Design review of the part built by this model. Coordinates are the model's own, in mm. A direction names the side the tool comes from. Give positions to 0.01 mm unless a question says otherwise; leave off trailing zeros. Write each loop counter-clockwise with the first axis right and the second up, starting at its lowest first coordinate (ties: lowest second). Pieces come first, ordered by that corner, then holes. Notation, with made-up numbers: M 78.25,-19.5 L 116.25,-19.5 A31 cw 116.25,19.5 Z; hole C 13,88.5 d3. An arc over 180 degrees is marked long. Answer in a Markdown table with one row per item.
```python
from build123d import *

# Parameters (mm, degrees)
SKETCH_1_R      = 1.1
SKETCH_1_R_2    = 1.6
EXTRUDE_1_DEPTH = 5


with BuildPart() as part:
    # ｽｹｯﾁ1 → ﾎﾞｽ - 押し出し1 (new body)
    with BuildSketch(Plane(origin=(0, 0, 0), x_dir=(1, 0, 0), z_dir=(0, 1, 0))):
        with BuildLine():
            Line((-15.999307359, 14.052631579), (-16.998961039, -23.921052632))
            ThreePointArc((-16.998961039, -23.921052632), (-16.149051198, -26.093222145), (-14, -27))
            Line((-14, -27), (14, -27))
            ThreePointArc((14, -27), (16.149051198, -26.093222145), (16.998961039, -23.921052632))
            Line((16.998961039, -23.921052632), (15.999307359, 14.052631579))
            ThreePointArc((15.999307359, 14.052631579), (15.39548143, 15.432700799), (14, 16))
            Line((14, 16), (-14, 16))
            ThreePointArc((-14, 16), (-15.39548143, 15.432700799), (-15.999307359, 14.052631579))
        make_face()
        with Locations(Location((-14, 14, 0), (0, 0, 270))):
            Circle(SKETCH_1_R, mode=Mode.SUBTRACT)
        with Locations(Location((14, 14, 0), (0, 0, 270))):
            Circle(SKETCH_1_R, mode=Mode.SUBTRACT)
        with Locations(Location((14, -14, 0), (0, 0, 270))):
            Circle(SKETCH_1_R, mode=Mode.SUBTRACT)
        with Locations(Location((-14, -14, 0), (0, 0, 270))):
            Circle(SKETCH_1_R, mode=Mode.SUBTRACT)
        with Locations(Location((-14, -24, 0), (0, 0, 270))):
            Circle(SKETCH_1_R_2, mode=Mode.SUBTRACT)
        with Locations(Location((14, -24, 0), (0, 0, 270))):
            Circle(SKETCH_1_R_2, mode=Mode.SUBTRACT)
        with BuildLine():
            Line((-14, 12), (-14, -12))
            ThreePointArc((-14, -12), (-12.585786438, -12.585786438), (-12, -14))
            Line((-12, -14), (12, -14))
            ThreePointArc((12, -14), (12.585786438, -12.585786438), (14, -12))
            Line((14, -12), (14, 12))
            ThreePointArc((14, 12), (12.585786438, 12.585786438), (12, 14))
            Line((12, 14), (-12, 14))
            ThreePointArc((-12, 14), (-12.585786438, 12.585786438), (-14, 12))
        make_face(mode=Mode.SUBTRACT)
    extrude(amount=EXTRUDE_1_DEPTH)


solid = part.part
```
1) To check wall thickness, follow probe 1 along X at (y, z) = (1.85, 24); probe 2 along Z at (x, y) = (4, 1.6); probe 3 along X at (y, z) = (4, 10). State the ranges of each line that lie inside material, in increasing order. Write a range as [from, to].
Geometry says:
| item | result |
|---|---|
| probe 1 | [-17, -15.6], [-12.4, 12.4], [15.6, 17] |
| probe 2 | [-16, -14], [14, 27] |
| probe 3 | [-16.63, -14], [14, 16.63] |
2) Add section C-C (y = 2.4). Write out the cut boundary in (x, z).
Geometry says:
| item | result |
|---|---|
| outline | M -17,23.92 L -16,-14.05 A2 ccw -14,-16 L 14,-16 A2 ccw 16,-14.05 L 17,23.92 A3 ccw 14,27 L -14,27 A3 ccw Z; hole C -14,24 d3.2; hole C -14,-14 d2.2; hole C -14,14 d2.2; hole M -14,-12 A2 cw -12,-14 L 12,-14 A2 cw 14,-12 L 14,12 A2 cw 12,14 L -12,14 A2 cw -14,12 Z; hole C 14,24 d3.2; hole C 14,-14 d2.2; hole C 14,14 d2.2 |
3) The part is to be moulded in two halves that separate along X. For faces 3 (the face through (0, 2, -16)), 4 (the face through (15.41, 2.46, -15.42)), 5 (the face through (-16.17, 2.46, 26.07)), 6 (the face through (-12.57, 2.46, -12.6)), say which applies: released by +X, released by -X, zero draft, split by the parting line, or undercut.
Geometry says:
| item | result |
|---|---|
| face 3 | zero draft |
| face 4 | released by +X |
| face 5 | released by -X |
| face 6 | undercut |
4) Add section A-A (x = -7.5). Write out the cut boundary in (y, z).
Geometry says:
| item | result |
|---|---|
| outline | M 0,-16 L 5,-16 L 5,-14 L 0,-14 Z; M 0,14 L 5,14 L 5,27 L 0,27 Z |
5) For faces 1 (the face through (0, 5, 15)), 2 (the face through (-14, 2, 0)), list the 3-axis set-ups (+Z, -Z, +X, -X, +Y, -Y) from which the entire face can be reached by the end or side of a thin tool; tool diameter is ignored.
Geometry says:
| item | result |
|---|---|
| face 1 | +Z, -Z, +X, -X, +Y |
| face 2 | +Y, -Y |
6) Add section B-B (z = 2.5). Write out the cut boundary in (x, y).
Geometry says:
| item | result |
|---|---|
| outline | M -16.44,0 L -14,0 L -14,5 L -16.44,5 Z; M 14,0 L 16.44,0 L 16.44,5 L 14,5 Z |
7) Insertion check: P1, Ø3.5, axis at x = 14, z = 14, coming from the +Y side; P2, Ø2, axis at y = 2.5, z = -11.5, coming from the +X side; P3, Ø1, axis at y = 3.5, z = 16.5, coming from the +X side; P4, Ø1.8, axis at x = -14, z = -14, coming from the -Y side. Each pin has a flat end and moves straight along its axis. Give the tip position at first contact, or say it passes through.
Geometry says:
| item | result |
|---|---|
| P1 | y = 5 |
| P2 | x = 16.09 |
| P3 | x = 16.82 |
| P4 | through |
